from build123d import *

# Parameters (mm, degrees)
BOSS_EXTRUDE1_DEPTH = 2.6
SKETCH2_W           = 23.9
SKETCH2_H           = 2
BOSS_EXTRUDE2_DEPTH = 5.85
CUT_EXTRUDE1_REACH  = 22.638
SKETCH3_R           = 1.6
BOSS_EXTRUDE3_DEPTH = 5.85
SKETCH5_W           = 1
SKETCH5_H           = 2.2
CUT_EXTRUDE2_DEPTH  = 2.1
SKETCH6_R           = 3.6
CUT_EXTRUDE3_DEPTH  = 1.5
FILLET1_R           = 0.5


with BuildPart() as part:
    # Sketch1 → Boss-Extrude1 (new body)
    with BuildSketch(Plane(origin=(0, 0, 0), x_dir=(1, 0, 0), z_dir=(0, 1, 0))):
        Polygon((-11.95, 12.45), (-11.95, -12.45), (11.95, -12.45), (11.95, 12.45), (4.95, 12.45), (4.95, 14.55), (-4.95, 14.55), (-4.95, 12.45), align=None)
    extrude(amount=BOSS_EXTRUDE1_DEPTH)

    # Sketch2 → Boss-Extrude2 (add)
    with BuildSketch(Plane.XZ):
        with Locations((0, 11.45)):
            Rectangle(SKETCH2_W, SKETCH2_H)
    extrude(amount=BOSS_EXTRUDE2_DEPTH)

    # Sketch3 → Cut-Extrude1 (cut, up to next)
    with BuildSketch(Plane(origin=(0, 2.6, 0), x_dir=(1, 0, 0), z_dir=(0, 1, 0)), mode=Mode.PRIVATE) as cut_extrude1_sk1:
        with Locations((-11.5, -7.45)):
            Circle(SKETCH3_R)
    cut_extrude1_tool1 = extrude(cut_extrude1_sk1.sketch, amount=-CUT_EXTRUDE1_REACH, mode=Mode.PRIVATE) & part.part
    # Sketch3 → Cut-Extrude1 (cut, up to next)
    with BuildSketch(Plane(origin=(0, 2.6, 0), x_dir=(1, 0, 0), z_dir=(0, 1, 0)), mode=Mode.PRIVATE) as cut_extrude1_sk2:
        with Locations((11.5, -7.45)):
            Circle(SKETCH3_R)
    cut_extrude1_tool2 = extrude(cut_extrude1_sk2.sketch, amount=-CUT_EXTRUDE1_REACH, mode=Mode.PRIVATE) & part.part
    add(cut_extrude1_tool1.solids().sort_by_distance((-11.5, 2.6, 7.45))[0], mode=Mode.SUBTRACT)
    add(cut_extrude1_tool2.solids().sort_by_distance((11.5, 2.6, 7.45))[0], mode=Mode.SUBTRACT)

    # Sketch4 → Boss-Extrude3 (add)
    with BuildSketch(Plane.XZ):
        with BuildLine():
            Line((-11.95, 5.914584747), (-11.95, 3.914584747))
            ThreePointArc((-11.95, 3.914584747), (-7.936061026, 7.45), (-11.95, 10.985415253))
            Line((-11.95, 10.985415253), (-11.95, 8.985415253))
            ThreePointArc((-11.95, 8.985415253), (-9.9, 7.45), (-11.95, 5.914584747))
        make_face()
        with BuildLine():
            Line((11.95, 10.985415253), (11.95, 8.985415253))
            ThreePointArc((11.95, 8.985415253), (9.9, 7.45), (11.95, 5.914584747))
            Line((11.95, 5.914584747), (11.95, 3.914584747))
            ThreePointArc((11.95, 3.914584747), (7.936061026, 7.45), (11.95, 10.985415253))
        make_face()
    extrude(amount=BOSS_EXTRUDE3_DEPTH)

    # Sketch5 → Cut-Extrude2 (cut)
    with BuildSketch(Plane.XZ.offset(5.85)):
        with Locations((-7.936061026, 7.45)):
            Rectangle(SKETCH5_W, SKETCH5_H)
    extrude(amount=-CUT_EXTRUDE2_DEPTH, mode=Mode.SUBTRACT)

    # Sketch6 → Cut-Extrude3 (cut)
    with BuildSketch(Plane(origin=(0, 2.6, 0), x_dir=(1, 0, 0), z_dir=(0, 1, 0))):
        with Locations((11.5, -7.45)):
            Circle(SKETCH6_R)
        with Locations((-11.5, -7.45)):
            Circle(SKETCH6_R)
    extrude(amount=-CUT_EXTRUDE3_DEPTH, mode=Mode.SUBTRACT)

    # Fillet1
    fillet1_edges = [part.edges().sort_by_distance(p)[0] for p in [
        (0, 2.6, 12.45),
        (0, 2.6, -14.55),
    ]]
    fillet(fillet1_edges, radius=FILLET1_R)


solid = part.part
Design review of the part built by this model. Coordinates are the model's own, in mm. A direction names the side the tool comes from. Round coordinates to 2 decimals unless told otherwise and drop trailing zeros. Order: outer loops, then holes, each group sorted by start corner. A loop starts at its lowest first (then second) coordinate and runs counter-clockwise, first axis right, second up. Notation, with made-up numbers: M 62,2.5 L 117,2.5 A15 ccw 117,6.5 Z; hole C 35.25,24 d4. An arc over 180 degrees is marked long. Answer as CSV lines item,"result". Start each with the question number.
1) Add section B-B (x = -3.25). Give the boundary of the cut face in (y, z), then the cut area to 3 significant figures.
2) Add section C-C (z = 7.45). Give the boundary of the cut face in (x, y), then the cut area to 3 significant figures.
3) Wall thickness on line 1 along Z through (x, y) = (-11.5, 0.4); line 2 along X through (y, z) = (-3.35, 7.45); line 3 along Z through (x, y) = (11.5, 1.85): over which ranges is each line inside the solid? List them lowest first. Write a range as [from, to].
4) Add section D-D (y = 1.5). Give the boundary of the cut face in (x, z), then the cut area to 3 significant figures.
5) Add section A-A (x = 11.5). Give the boundary of the cut face in (y, z), then the cut area to 3 significant figures.
6) Tool access review of faces 1 (the face through (-11.95, -2, 11)), 2 (the face through (0, 1, -14.55)), 3 (the face through (-8, 1, -12.45)), 4 (the face through (8, 1, -12.45)), 5 (the face through (-7.9, 1.9, 7.5)): name each direction out of +Z, -Z, +X, -X, +Y, -Y from which nothing blocks a thin tool from reaching the whole face with its end or side.
7) The part is to be moulded in two halves that separate along X. For faces 6 (the face through (-8.174, -2.884, 6.17)), 7 (the face through (11.95, 0.3, -1.4)), 8 (the face through (0, -2, 12.45)), say which applies: +X half, -X half, draft (parallel to the pull), parting line (faces both ways), or undercut.
8) For pin 1 Ø1.7 at (y, z) = (1.5, -13.5) entering from +X; pin 2 Ø4 at (y, z) = (1.5, 8.5) entering from +X; pin 3 Ø6 at (x, z) = (-7.5, -6.5) entering from -Y; pin 4 Ø1.2 at (x, z) = (-10, 6) entering from +Y, all flat-tipped, find the tip position at first contact; note any pin that passes through.
Resolved:
1,outline,"M -5.85,10.45 L 0,10.45 L 0,-14.55 L 2.1,-14.55 A0.5 ccw 2.6,-14.05 L 2.6,11.95 A0.5 ccw 2.1,12.45 L -5.85,12.45 Z"
1,area,"81.8 mm^2"
2,outline,"M -9.9,-5.85 L -8.44,-5.85 L -8.44,-3.75 L -7.94,-3.75 L -7.94,0 L 7.94,0 L 7.94,-5.85 L 9.9,-5.85 L 9.9,1.1 L 7.9,1.1 L 7.9,2.6 L -7.9,2.6 L -7.9,1.1 L -9.9,1.1 Z"
2,area,"67.4 mm^2"
3,line 1,"[-12.45, 5.85], [9.05, 12.45]"
3,line 2,"[-9.9, -7.94], [7.94, 9.9]"
3,line 3,"[-12.45, 3.85], [11.05, 12.45]"
4,outline,"M -11.95,-12.45 L -4.95,-12.45 L -4.95,-14.55 L 4.95,-14.55 L 4.95,-12.45 L 11.95,-12.45 L 11.95,3.88 A3.6 cw long 11.95,11.02 L 11.95,12.45 L -11.95,12.45 L -11.95,11.02 A3.6 cw long -11.95,3.88 Z"
4,area,"569 mm^2"
5,outline,"M -5.85,3.89 L 0,3.89 L 0,-12.45 L 2.6,-12.45 L 2.6,3.85 L 1.1,3.85 L 1.1,5.85 L -5.85,5.85 Z; M -5.85,9.05 L 1.1,9.05 L 1.1,11.05 L 2.6,11.05 L 2.6,11.95 A0.5 ccw 2.1,12.45 L -5.85,12.45 Z"
5,area,"81.7 mm^2"
6,face 1,"+Z, -Z, -X, +Y, -Y"
6,face 2,"-Z, +X, -X, +Y, -Y"
6,face 3,"-Z, -X, +Y, -Y"
6,face 4,"-Z, +X, +Y, -Y"
6,face 5,"+Y"
7,face 6,"undercut"
7,face 7,"+X half"
7,face 8,"draft"
8,pin 1,"x = 4.95"
8,pin 2,"x = 11.95"
8,pin 3,"y = 0"
8,pin 4,"y = 1.1"
